```python
from build123d import *

# Parameters (mm, degrees)
BOSS_EXTRUDE1_DEPTH = 25.4
SKETCH2_R           = 12.6
SKETCH2_R_2         = 8.6
BOSS_EXTRUDE2_DEPTH = 6
CUT_EXTRUDE1_DEPTH  = 6
FILLET1_R           = 1


with BuildPart() as part:
    # Sketch1 → Boss-Extrude1 (new body)
    with BuildSketch(Plane.XY):
        Polygon((-10.189534884, 0), (-10.189534884, 9), (15.210465116, 9), (15.210465116, 0), (21.210465116, 0), (21.210465116, 18.375), (-16.189534884, 18.375), (-16.189534884, 0), align=None)
    extrude(amount=BOSS_EXTRUDE1_DEPTH)

    # Sketch2 → Boss-Extrude2 (add)
    with BuildSketch(Plane(origin=(0, 18.375, 0), x_dir=(1, 0, 0), z_dir=(0, 1, 0))):
        with Locations((2.510465116, -12.7)):
            Circle(SKETCH2_R)
        with Locations((2.510465116, -12.7)):
            Circle(SKETCH2_R_2, mode=Mode.SUBTRACT)
    extrude(amount=BOSS_EXTRUDE2_DEPTH)

    # Sketch3 → Cut-Extrude1 (cut)
    with BuildSketch(Plane(origin=(0, 24.375, 0), x_dir=(1, 0, 0), z_dir=(0, 1, 0))):
        with BuildLine():
            ThreePointArc((-1.789534884, -5.252181527), (0.284621328, -4.393037894), (2.510465116, -4.1))
            Line((2.510465116, -4.1), (2.510465116, -0.1))
            ThreePointArc((2.510465116, -0.1), (-0.750654852, -0.529334589), (-3.789534884, -1.788079912))
            Line((-3.789534884, -1.788079912), (-1.789534884, -5.252181527))
        make_face()
        with BuildLine():
            Line((2.510465116, -0.1), (2.510465116, -4.1))
            ThreePointArc((2.510465116, -4.1), (4.736308904, -4.393037894), (6.810465116, -5.252181527))
            Line((6.810465116, -5.252181527), (8.810465116, -1.788079912))
            ThreePointArc((8.810465116, -1.788079912), (5.771585085, -0.529334589), (2.510465116, -0.1))
        make_face()
    extrude(amount=-CUT_EXTRUDE1_DEPTH, mode=Mode.SUBTRACT)

    # Fillet1
    fillet1_edges = [part.edges().sort_by_distance(p)[0] for p in [
        (2.510465116, 24.375, 21.3),
    ]]
    fillet(fillet1_edges, radius=FILLET1_R)


solid = part.part
```
Verification items for the finished model (mm, model axes). A direction names the side the tool comes from. Coordinates: 2 decimals unless noted, no trailing zeros. Write each loop counter-clockwise with the first axis right and the second up, starting at its lowest first coordinate (ties: lowest second). Pieces come first, ordered by that corner, then holes. Notation, with made-up numbers: M -28,86 L 15,86 A12 ccw 15,100 Z; hole C 14.25,77 d8. An arc over 180 degrees is marked long. Answer as a JSON object with one key per item and string values. Group by question number.
(1) Material ranges on line 1 (X direction, y = 21.3, z = 12.7); line 2 (Y direction, x = -10.5, z = 9.5) (3 decimals); line 3 (Y direction, x = -8, z = 20.75) (3 decimals), recorded low to high.
(2) Tool access check on faces 4 (the face through (2, 11, 25.4)), 5 (the face through (-10.19, 4, 13)), 6 (the face through (2.195, 20.84, 21.294)), 7 (the face through (-2.8, 21.4, 3.5)). Record the directions out of +Z, -Z, +X, -X, +Y, -Y that give a thin tool (end or side, any length) a straight path to the whole face; none if there is none.
(3) Cross-section at C-C, the plane x = 16. Record the cut outline in (y, z) (3 decimals), and give its area (3 significant figures).
(4) Release check for a two-part mould opening along X. For faces 1 (the face through (21.21, 9, 13)), 2 (the face through (7.8, 21.42, 3.54)), 3 (the face through (18, 0, 13)) record: +X half, -X half, draft (parallel to the pull), parting line (faces both ways), or undercut.
(5) Cross-section at D-D, the plane y = 21. Record the cut outline in (x, z).
(6) Cross-section at B-B, the plane z = 12.7. Record the cut outline in (x, y) (3 decimals), and give its area (3 significant figures).
(7) Cross-section at A-A, the plane y = 6. Record the cut outline in (x, z).
(8) Gauge pin test, flat end, axial feed: pin 1 (10.5 mm diameter, centred on x = 2.51, z = 12.7, fed in from +Y) (3 decimals). Record the tip position at first contact, or that the pin passes through.
Reply:
{
 "1": {"line 1": "-10.09 to -6.09, 11.11 to 15.11", "line 2": "0 to 18.375", "line 3": "9 to 18.375"},
 "2": {"face 4": "+Z, +X, -X, +Y, -Y", "face 5": "+Z, -Z, -Y", "face 6": "+Y", "face 7": "-Z, +Y"},
 "3": {"outline": "M 0,0 L 18.375,0 L 18.375,25.4 L 0,25.4 Z", "area": "467 mm²"},
 "4": {"face 1": "+X half", "face 2": "undercut", "face 3": "draft"},
 "5": {"outline": "M -3.79,1.79 L -1.79,5.25 A8.6 cw long 6.81,5.25 L 8.81,1.79 A12.6 ccw long Z"},
 "6": {"outline": "M -16.19,0 L -10.19,0 L -10.19,9 L 15.21,9 L 15.21,0 L 21.21,0 L 21.21,18.375 L 15.11,18.375 L 15.11,24.375 L 12.11,24.375 A1 ccw 11.11,23.375 L 11.11,18.375 L -6.09,18.375 L -6.09,23.375 A1 ccw -7.09,24.375 L -10.09,24.375 L -10.09,18.375 L -16.19,18.375 Z", "area": "506 mm²"},
 "7": {"outline": "M -16.19,0 L -10.19,0 L -10.19,25.4 L -16.19,25.4 Z; M 15.21,0 L 21.21,0 L 21.21,25.4 L 15.21,25.4 Z"},
 "8": {"pin 1": "y = 18.375"}
}
